Autodesk Inventor part; units mm, degrees
ref_plane "YZ Plane" through (0, 0, 0) normal (1, 0, 0) x (0, 1, 0)
ref_plane "XZ Plane" through (0, 0, 0) normal (0, 1, 0) x (-1, 0, 0)
ref_plane "XY Plane" through (0, 0, 0) normal (0, 0, 1) x (1, 0, 0)
sketch "Sketch11" plane through (0, 0, 0) normal (0, 1, 0) x (-1, 0, 0)
  line L0 (0, 0) -> (52.5, 0)
  line L1 (52.5, 0) -> (52.5, 32)
  line L2 (52.5, 32) -> (0, 32)
  line L3 (0, 32) -> (0, 0)
  line L4 (52.5, 32) -> (49.5, 32)
  dimension "d63" = 52.5
  dimension "d64" = 32
  dimension "d67" = 3
extrude "Extrusion10" add sketch "Sketch11" along normal blind 6
sketch "Sketch12" plane through (0, 0, 0) normal (0, -1, 0) x (1, 0, 0)
  line L0 (-52.5, 32) -> (-49.5, 32)
  line L1 (-52.5, 32) -> (0, 32)
  line L2 (-49.5, 32) -> (-49.5, 26)
  circle A0 centre (-49.5, 26) radius 2.25
  circle A1 centre (-3, 26) radius 2.25
  circle A2 centre (-49.5, 6) radius 2.25
  circle A3 centre (-3, 6) radius 2.25
  point P0 (0, 0)
  dimension "d68" = 3
  dimension "d69" = 6
  dimension "d70" = 4.5
  dimension "d73" = 46.5
  dimension "d76" = 20
extrude "Extrusion11" cut sketch "Sketch12" against normal blind 10
properties part number "suporte-barra" material "Steel, Carbon"
Build history of the part. All positions in model axes, mm. Coordinates: 2 decimals unless noted, no trailing zeros. Order: outer loops, then holes, each group sorted by start corner. A loop starts at its lowest first (then second) coordinate and runs counter-clockwise, first axis right, second up. Notation, with made-up numbers: (53, 40) - (78, 40) arc R9 cw to (78, 55) - close; hole circle Ø8 at (-36, 64.5). An arc over 180 degrees is marked (long way). Put each result on its own line as item: value.
1. Saw through at C-C (y = 4.8). Write the cut outline in (x, z).
Answer sheet:
outline: (-52.5, 0) - (0, 0) - (0, 32) - (-52.5, 32) - close; hole circle Ø4.5 at (-49.5, 6); hole circle Ø4.5 at (-49.5, 26); hole circle Ø4.5 at (-3, 6); hole circle Ø4.5 at (-3, 26)
2. Pull direction X, two halves, no side cores. Call faces 1 (the face through (-27, 3, 32)), 2 (the face through (-52.5, 3, 16)), 3 (the face through (-3.488, 2.958, 23.804)): pulls with the +X half, pulls with the -X half, needs draft (parallel to the pull), parting line crosses it, or undercut.
Answer sheet:
face 1: needs draft
face 2: pulls with the -X half
face 3: undercut
3. Saw through at A-A (z = 26). Write the cut outline in (x, y).
Answer sheet:
outline: (-52.5, 0) - (-51.75, 0) - (-51.75, 6) - (-52.5, 6) - close; (-47.25, 0) - (-5.25, 0) - (-5.25, 6) - (-47.25, 6) - close; (-0.75, 0) - (0, 0) - (0, 6) - (-0.75, 6) - close
4. Saw through at B-B (x = -49.5). Write the cut outline in (y, z), and give its area (3 significant figures).
Answer sheet:
outline: (0, 0) - (6, 0) - (6, 3.75) - (0, 3.75) - close; (0, 8.25) - (6, 8.25) - (6, 23.75) - (0, 23.75) - close; (0, 28.25) - (6, 28.25) - (6, 32) - (0, 32) - close
area: 138 mm^2
5. Probe line 1 along Z through (x, y) = (-49.5, 3.5); line 2 along X through (y, z) = (2.25, 28); line 3 along X through (y, z) = (1.95, 5.5). List the from-to ranges inside material, lowest first. Write a range as [from, to].
Answer sheet:
line 1: z = [0, 3.75], [8.25, 23.75], [28.25, 32]
line 2: x = [-52.5, -50.53], [-48.47, -4.03], [-1.97, 0]
line 3: x = [-52.5, -51.69], [-47.31, -5.19], [-0.81, 0]
